Could you check a few things on this model? Use its own coordinates, in mm. Face numbers are marked on the shaded views. A direction names the side the tool comes from. Give positions to 0.01 mm unless a question says otherwise; leave off trailing zeros. Order: outer loops, then holes, each group sorted by start corner. A loop starts at its lowest first (then second) coordinate and runs counter-clockwise, first axis right, second up. Notation, with made-up numbers: M 38.5,52.5 L 45.5,52.5 A29 cw 45.5,83.5 Z; hole C 58.5,-10 d1. An arc over 180 degrees is marked long. Return JSON: item names as keys, results as strings. Group by question number.
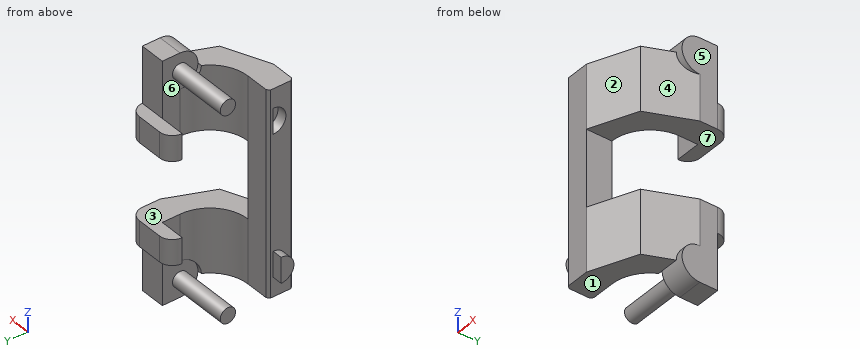
```python
from build123d import *

# Parameters (mm, degrees)
BOSS_EXTRUDE1_DEPTH   = 10
BOSS_EXTRUDE1_2_DEPTH = 10
BOSS_EXTRUDE2_START   = -7
BOSS_EXTRUDE2_DEPTH   = 80
CUT_EXTRUDE1_START    = 2
CUT_EXTRUDE1_DEPTH    = 2
SKETCH9_W             = 80
SKETCH9_H             = 10
BOSS_EXTRUDE4_DEPTH   = 10
CUT_EXTRUDE3_DEPTH    = 80
CUT_EXTRUDE4_START    = -32
CUT_EXTRUDE4_DEPTH    = 30
SKETCH7_R             = 3
BOSS_EXTRUDE5_DEPTH   = 24
BOSS_EXTRUDE6_DEPTH   = 10
BOSS_EXTRUDE8_START   = 10
BOSS_EXTRUDE8_DEPTH   = 10
BOSS_EXTRUDE3_DEPTH   = 4
CUT_EXTRUDE5_DEPTH    = 4


with BuildPart() as part:
    # Sketch3 → Boss-Extrude1 (new body)
    with BuildSketch(Plane(origin=(0, 0, 0), x_dir=(0, 0, -1), z_dir=(1, 0, 0))):
        with BuildLine():
            Line((-47, 7), (-47, 0))
            ThreePointArc((-47, 0), (-40, -7), (-33, 0))
            Line((-33, 0), (-15, 0))
            Line((-15, 0), (-15, 7))
            Line((-15, 7), (-47, 7))
        make_face()
    extrude(amount=BOSS_EXTRUDE1_DEPTH)

    # Sketch5 → Boss-Extrude2 (add)
    with BuildSketch(Plane(origin=(0, 0, -47), x_dir=(-1, 0, 0), z_dir=(0, 0, -1)).offset(BOSS_EXTRUDE2_START)):
        with BuildLine():
            Line((-10, 0), (0, 0))
            ThreePointArc((0, 0), (4.393398282, -10.606601718), (15, -15))
            Line((15, -15), (15, -25))
            Line((15, -25), (-2.67766953, -17.67766953))
            Line((-2.67766953, -17.67766953), (-10, 0))
        make_face()
    extrude(amount=-BOSS_EXTRUDE2_DEPTH)

    # Sketch6 → Cut-Extrude1 (cut)
    with BuildSketch(Plane.ZY.offset(CUT_EXTRUDE1_START)):
        with BuildLine():
            Line((-33, 0), (-40, 0))
            Line((-40, 0), (-40, -7))
            ThreePointArc((-40, -7), (-35.050252532, -4.949747468), (-33, 0))
        make_face()
        with BuildLine():
            Line((40, 0), (33, 0))
            ThreePointArc((33, 0), (35.050252532, -4.949747468), (40, -7))
            Line((40, -7), (40, 0))
        make_face()
    extrude(amount=-CUT_EXTRUDE1_DEPTH, mode=Mode.SUBTRACT)

    # Sketch9 → Boss-Extrude4 (add)
    with BuildSketch(Plane.ZY.offset(15)):
        with Locations((0, -20)):
            Rectangle(SKETCH9_W, SKETCH9_H)
    extrude(amount=BOSS_EXTRUDE4_DEPTH)

    # Sketch10 → Cut-Extrude3 (cut)
    with BuildSketch(Plane(origin=(0, 0, -40), x_dir=(-1, 0, 0), z_dir=(0, 0, -1))):
        Polygon((25, -15), (24, -15), (25, -16), align=None)
        Polygon((25, -25), (24, -25), (25, -24), align=None)
    extrude(amount=-CUT_EXTRUDE3_DEPTH, mode=Mode.SUBTRACT)

    # Sketch5<3> → Cut-Extrude4 (cut)
    with BuildSketch(Plane(origin=(0, 0, -47), x_dir=(-1, 0, 0), z_dir=(0, 0, -1)).offset(CUT_EXTRUDE4_START)):
        with BuildLine():
            Line((0, 0), (-10, 0))
            Line((-10, 0), (-2.67766953, -17.67766953))
            Line((-2.67766953, -17.67766953), (15, -25))
            Line((15, -25), (15, -15))
            ThreePointArc((15, -15), (4.393398282, -10.606601718), (0, 0))
        make_face()
    extrude(amount=-CUT_EXTRUDE4_DEPTH, mode=Mode.SUBTRACT)



with BuildPart() as body_2:
    # Sketch3 → Boss-Extrude1 2 (new body)
    with BuildSketch(Plane(origin=(0, 0, 0), x_dir=(0, 0, -1), z_dir=(1, 0, 0))):
        with BuildLine():
            Line((15, 7), (15, 0))
            Line((15, 0), (33, 0))
            ThreePointArc((33, 0), (40, -7), (47, 0))
            Line((47, 0), (47, 7))
            Line((47, 7), (15, 7))
        make_face()
    extrude(amount=BOSS_EXTRUDE1_2_DEPTH)


with BuildPart() as part_1:
    add(part.part)

    add(body_2.part)  # Boss-Extrude5 merges body 2
    # Sketch7 → Boss-Extrude5 (add)
    with BuildSketch(Plane.ZY):
        with Locations((-40, 0)):
            Circle(SKETCH7_R)
        with Locations(Location((40, 0, 0), (0, 0, 180))):
            Circle(SKETCH7_R)
    extrude(amount=BOSS_EXTRUDE5_DEPTH)

    # Sketch11 → Boss-Extrude6 (add)
    with BuildSketch(Plane.XY.offset(-15)):
        with BuildLine():
            Line((-10, 7), (0, 7))
            Line((0, 7), (10, 7))
            ThreePointArc((10, 7), (8.535533906, 10.535533906), (5, 12))
            Line((5, 12), (-5, 12))
            ThreePointArc((-5, 12), (-8.535533906, 10.535533906), (-10, 7))
        make_face()
    extrude(amount=-BOSS_EXTRUDE6_DEPTH)

    # Sketch13 → Boss-Extrude8 (add)
    with BuildSketch(Plane.XY.offset(15).offset(BOSS_EXTRUDE8_START)):
        with BuildLine():
            Line((-10, 7), (0, 7))
            Line((0, 7), (10, 7))
            ThreePointArc((10, 7), (8.535533906, 10.535533906), (5, 12))
            Line((5, 12), (-5, 12))
            ThreePointArc((-5, 12), (-8.535533906, 10.535533906), (-10, 7))
        make_face()
    extrude(amount=-BOSS_EXTRUDE8_DEPTH)

    # Sketch8 → Boss-Extrude3 (add)
    with BuildSketch(Plane.ZY.offset(25)):
        with BuildLine():
            Line((-32.5, -17), (-22.5, -17))
            ThreePointArc((-22.5, -17), (-27.5, -22), (-32.5, -17))
        make_face()
    extrude(amount=BOSS_EXTRUDE3_DEPTH)

    # Sketch8<4> → Cut-Extrude5 (cut)
    with BuildSketch(Plane.ZY.offset(25)):
        with BuildLine():
            Line((32.5, -17), (22.5, -17))
            ThreePointArc((22.5, -17), (27.5, -22), (32.5, -17))
        make_face()
    extrude(amount=-CUT_EXTRUDE5_DEPTH, mode=Mode.SUBTRACT)


solid = part_1.part
```
1. Imagine slicing it at D-D, the plane x = -12. Please give me the cut outline in (y, z), plus the area to 3 significant figures.
2. Imagine slicing it at A-A, the plane x = -7. Please give me the cut outline in (y, z), plus the area to 3 significant figures.
3. Imagine slicing it at C-C, the plane y = -12. Please give me the cut outline in (x, z), plus the area to 3 significant figures.
4. Imagine slicing it at B-B, the plane z = 27.5. Please give me the cut outline in (x, y), plus the area to 3 significant figures.
5. For pin 1 (2 mm diameter, centred on x = -0.5, z = 17.5, fed in from -Y); pin 2 (8 mm diameter, centred on x = -3, z = -19, fed in from -Y); pin 3 (6 mm diameter, centred on x = 2, z = 11.5, fed in from -Y); pin 4 (10 mm diameter, centred on x = -21.5, z = -13.5, fed in from +Y), each with a flat end and sliding along its axis, tell me the tip position at first contact or that it passes through.
6. I need wall thicknesses on L1, parallel to Z at x = 4, y = 10.5; L2, parallel to Z at x = -9.5, y = -19.5; L3, parallel to Y at x = -24, z = -18.5. Which ranges of each line are inside material? Lowest first, please. Write a range as from..to.
7. Which directions (+Z, -Z, +X, -X, +Y, -Y) give clear straight access to the entire face, cutting with the end or side of a thin tool? Please do the marked faces 4, 5, 6 and 7.
8. If we mould it in two halves opening along Z, with no side actions, what happens to the marked faces 1, 2 and 3? For each: pulls with the +Z half, pulls with the -Z half, needs draft (parallel to the pull), parting line crosses it, or undercut.
Values:
{
 "1": {"outline": "M -23.76,-40 L -14.7,-40 L -14.7,-15 L -23.76,-15 Z; M -23.76,15 L -14.7,15 L -14.7,40 L -23.76,40 Z; C 0,-40 d6; C 0,40 d6", "area": "510 mm²"},
 "2": {"outline": "M -21.69,-40 L -12.69,-40 L -12.69,-15 L -21.69,-15 Z; M -21.69,15 L -12.69,15 L -12.69,40 L -21.69,40 Z; C 0,-40 d6; C 0,40 d6; M 7,-25 L 11.58,-25 L 11.58,-15 L 7,-15 Z; M 7,15 L 11.58,15 L 11.58,25 L 7,25 Z", "area": "598 mm²"},
 "3": {"outline": "M -6,-40 L 5.03,-40 L 5.03,-15 L -6,-15 Z; M -6,15 L 5.03,15 L 5.03,40 L -6,40 Z", "area": "551 mm²"},
 "4": {"outline": "M -25,-24 L -24,-25 L -15,-25 L 2.68,-17.68 L 10,0 L 10,7 L 0,7 L 0,0 A15 cw -15,-15 L -24,-15 L -25,-16 L -25,-17 L -21,-17 L -21,-22 L -25,-22 Z", "area": "414 mm²"},
 "5": {"pin 1": "stops at y = -19.41", "pin 2": "stops at y = -21.69", "pin 3": "passes through", "pin 4": "stops at y = -15"},
 "6": {"L1": "z = -25..-15, 15..25", "L2": "z = -40..-15, 15..40", "L3": "y = -25..-15"},
 "7": {"face 4": "+X, -Y", "face 5": "+Z, -Z, +X, +Y, -Y", "face 6": "-X", "face 7": "+X, +Y, -Y"},
 "8": {"face 1": "pulls with the -Z half", "face 2": "needs draft", "face 3": "undercut"}
}
